from build123d import *

# Parameters (mm, degrees)
F1_DEPTH = 127
F3_DEPTH = 76.2
F4_SIZE2 = 101.6
F4_SIZE  = 76.2
F5_R     = 5.08
F6_R     = 15.24
F7_DEPTH = 50.8
F8_R     = 19.05
F9_DEPTH = 127


with BuildPart() as f1:
    # F0 (on Front) → F1 (new body)
    with BuildSketch(Plane.XZ):
        Polygon((101.6, -63.5), (101.6, 63.5), (0, 63.5), (0, 0), (-38.1, 0), (-38.1, -63.5), align=None)
        Polygon((0, 0), (0, 63.5), (-101.6, 63.5), (-101.6, -63.5), (-38.1, -63.5), (-38.1, 0), align=None)
    extrude(amount=F1_DEPTH)

    # F2 (on face) → F3 (cut)
    with BuildSketch(Plane.XZ.offset(127)):
        Polygon((-38.1, 0), (-38.1, -63.5), (101.6, -63.5), (101.6, 63.5), (0, 63.5), (0, 0), align=None)
    extrude(amount=-F3_DEPTH, mode=Mode.SUBTRACT)

    # F4
    f4_edges = [f1.edges().sort_by_distance(p)[0] for p in [
        (101.6, -25.4, 63.5),
    ]]
    f4_side = f1.faces().sort_by_distance((-21.771429, -52.614286, 63.5))[0]
    chamfer(f4_edges, length=F4_SIZE, length2=F4_SIZE2, reference=f4_side)

    # F5
    f5_edges = [f1.edges().sort_by_distance(p)[0] for p in [
        (63.5, -50.8, 12.7),
        (63.5, 0, 12.7),
        (12.7, -50.8, 63.5),
        (0, -88.9, 63.5),
        (-50.8, -127, 63.5),
        (0, -127, 31.75),
        (0, -88.9, 0),
        (31.75, -50.8, -63.5),
        (101.6, -50.8, -50.8),
        (101.6, -25.4, -63.5),
        (-101.6, -127, 0),
        (-69.85, -127, -63.5),
        (-38.1, 0, 63.5),
        (-101.6, 0, 0),
        (0, 0, -63.5),
        (-101.6, -63.5, -63.5),
        (-38.1, -88.9, -63.5),
        (-101.6, -63.5, 63.5),
        (-38.1, -127, -31.75),
        (-19.05, -127, 0),
        (-38.1, -88.9, 0),
        (-19.05, -50.8, 0),
        (-38.1, -50.8, -31.75),
        (0, -50.8, 31.75),
    ]]
    fillet(f5_edges, radius=F5_R)

    # F6 (on face) → F7 (cut, through all)
    with BuildSketch(Plane.XZ.offset(50.8)):
        with Locations((12.7, -17.78)):
            Circle(F6_R)
    extrude(amount=-F7_DEPTH, mode=Mode.SUBTRACT)

    # F8 (on face) → F9 (cut, through all)
    with BuildSketch(Plane.XY.offset(63.5)):
        with Locations((-60.7483349741, -66.2939995527)):
            Circle(F8_R)
    extrude(amount=-F9_DEPTH, mode=Mode.SUBTRACT)


solid = f1.part
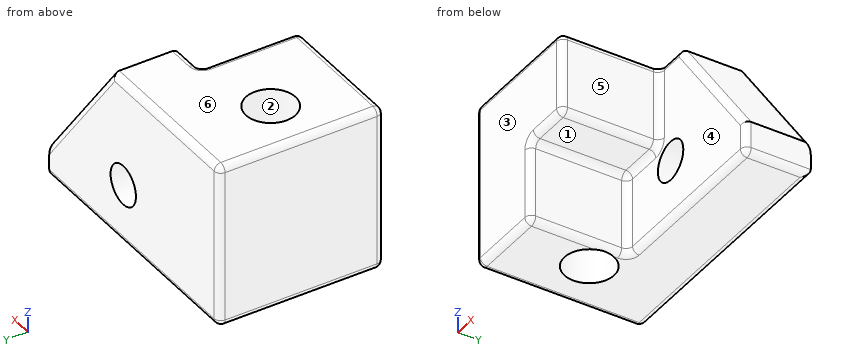
The listing builds one solid part. Answer for the finished solid, in the listing's coordinates (mm). Face numbers are marked on the shaded views. A direction names the side the tool comes from. Give positions to 0.01 mm unless a question says otherwise; leave off trailing zeros. Write each loop counter-clockwise with the first axis right and the second up, starting at its lowest first coordinate (ties: lowest second). Pieces come first, ordered by that corner, then holes.
1) Given P1, Ø8, axis at x = -21, y = -102.5, coming from the -Z side; P2, Ø1.5, axis at x = -47, y = -78, coming from the -Z side, each flat-ended and moving along its own axis, determine where each tip first touches the part or whether it passes through.
2) Section B-B (y = -101.5) is taken. Write down the section's boundary in (x, z), and give its area (3 significant figures).
3) A tool of negligible diameter and unlimited length cuts with its end or side. For the marked faces 4, 5 and 6, from which of +Z, -Z, +X, -X, +Y, -Y can it reach the whole face along a straight path? Write none if from no direction.
4) For a pull along Y with two mould halves and no side action, classify the marked faces 1, 2 and 3 as pulls with the +Y half, pulls with the -Y half, needs draft (parallel to the pull), parting line crosses it, or undercut.
5) Section A-A (x = 12.7) is taken. Write down the section's boundary in (y, z), and give its area (3 significant figures).
6) Section C-C (y = -26) is taken. Write down the section's boundary in (x, z), and give its area (3 significant figures).
7) Find the intervals of material crossed by L1, parallel to Z at x = 12.7, y = -32; L2, parallel to X at y = -67, z = 48.5; L3, parallel to Y at x = 42, z = -5, in increasing order.
8) Section D-D (x = -17) is taken. Write down the section's boundary in (y, z).
Response:
1. P1: stops at z = 0
1. P2: passes through
2. outline: (-101.6, -58.42) arc R5.08 ccw to (-96.52, -63.5) - (-43.18, -63.5) arc R5.08 ccw to (-38.1, -58.42) - (-38.1, -5.08) arc R5.08 cw to (-33.02, 0) - (-5.08, 0) arc R5.08 ccw to (0, 5.08) - (0, 58.42) arc R5.08 ccw to (-5.08, 63.5) - (-96.52, 63.5) arc R5.08 ccw to (-101.6, 58.42) - close
2. area: 10,500 mm2
3. face 4: -Z, +X, -Y
3. face 5: +Z, -Z, +X, -Y
3. face 6: +Z, +X, -X, +Y, -Y
4. face 1: needs draft
4. face 2: undercut
4. face 3: pulls with the -Y half
5. outline: (-50.8, -58.42) arc R5.08 ccw to (-45.72, -63.5) - (-5.08, -63.5) arc R5.08 ccw to (0, -58.42) - (0, -33.02) - (-50.8, -33.02) - close; (-50.8, -2.54) - (0, -2.54) - (0, 58.42) arc R5.08 ccw to (-5.08, 63.5) - (-45.72, 63.5) arc R5.08 ccw to (-50.8, 58.42) - close
5. area: 4,880 mm2
6. outline: (-101.6, -58.42) arc R5.08 ccw to (-96.52, -63.5) - (96.52, -63.5) arc R5.08 ccw to (101.6, -58.42) - (101.6, -38.1) - (25.4, 63.5) - (-96.52, 63.5) arc R5.08 ccw to (-101.6, 58.42) - close; hole circle Ø30.48 at (12.7, -17.78)
6. area: 21,200 mm2
7. L1: z = -63.5 to -33.02, -2.54 to 63.5
7. L2: x = -101.6 to -79.79, -41.71 to 0
7. L3: y = -50.8 to 0
8. outline: (-127, 5.08) arc R5.08 ccw to (-121.92, 0) - (-55.88, 0) arc R5.08 cw to (-50.8, -5.08) - (-50.8, -58.42) arc R5.08 ccw to (-45.72, -63.5) - (-5.08, -63.5) arc R5.08 ccw to (0, -58.42) - (0, 58.42) arc R5.08 ccw to (-5.08, 63.5) - (-121.92, 63.5) arc R5.08 ccw to (-127, 58.42) - close
